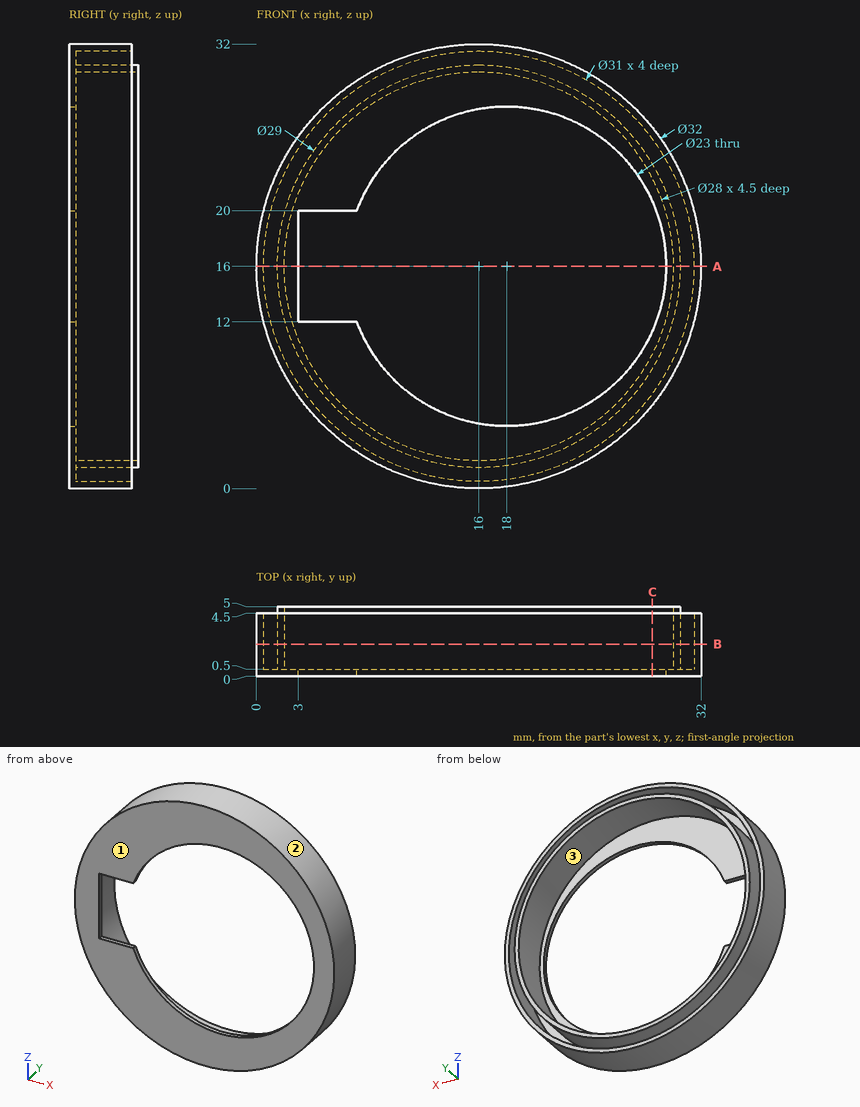
Design review of the part shown in the three views and the two pictorial views. Dimensions are in mm from the part's minimum x, y and z. Give positions to 0.01 mm unless a question says otherwise; leave off trailing zeros. Loops run counter-clockwise (first coordinate to the right, second up) from the corner with the lowest first, then second, coordinate; pieces in that order, holes last. Notation, with made-up numbers: M 12,58 L 19,58 A28 cw 19,79 Z; hole C 74,17 d5. An arc over 180 degrees is marked long. Put each result on its own line as item: value. Start each with the question number.
(1) Add section C-C, the plane x = 28.5. Write out the cut boundary in (y, z).
(2) For pin 1 (3 mm diameter, centred on x = 4, z = 19.5, fed in from -Y); pin 2 (1.5 mm diameter, centred on x = 28, y = 3.5, fed in from +Z); pin 3 (3 mm diameter, centred on y = 2.5, z = 18.5, fed in from -X), all flat-tipped, find the tip position at first contact; note any pin that passes through.
(3) Add section B-B, the plane y = 2.3. Write out the cut boundary in (x, z).
(4) The part is to be moulded in two halves that separate along Z. For the marked faces 1, 2 and 3, say which applies: +Z half, -Z half, draft (parallel to the pull), parting line (faces both ways), or undercut.
(5) Add section A-A, the plane z = 16. Write out the cut boundary in (x, y), then the cut area to 4 significant figures.
(6) Wall thickness on L1, parallel to X at y = 3.4, z = 16; L2, parallel to Z at x = 16.5, y = 0.8; L3, parallel to Z at x = 21, y = 1.55: over which ranges is each line inside the solid? List them lowest first.
Result:
1. outline: M 0,6.01 L 4.5,6.01 L 4.5,6.83 L 0.5,6.83 L 0.5,8.65 L 5,8.65 L 5,9.7 L 0.5,9.7 L 0.5,11.31 L 0,11.31 Z; M 0,20.69 L 0.5,20.69 L 0.5,22.3 L 5,22.3 L 5,23.35 L 0.5,23.35 L 0.5,25.17 L 4.5,25.17 L 4.5,25.99 L 0,25.99 Z
2. pin 1: stops at y = 0
2. pin 2: stops at z = 27.38
2. pin 3: stops at x = 0.03
3. outline: C 16,16 d32; C 16,16 d29; hole C 16,16 d31; hole C 16,16 d28
4. face 1: draft
4. face 2: parting line
4. face 3: undercut
5. outline: M 0,0 L 3,0 L 3,0.5 L 2,0.5 L 2,5 L 1.5,5 L 1.5,0.5 L 0.5,0.5 L 0.5,4.5 L 0,4.5 Z; M 29.5,0 L 32,0 L 32,4.5 L 31.5,4.5 L 31.5,0.5 L 30.5,0.5 L 30.5,5 L 30,5 L 30,0.5 L 29.5,0.5 Z
5. area: 11.25 mm^2
6. L1: x = 0 to 0.5, 1.5 to 2, 30 to 30.5, 31.5 to 32
6. L2: z = 0.01 to 0.51, 1.51 to 2.01, 29.99 to 30.49, 31.49 to 31.99
6. L3: z = 0.8 to 1.33, 2.39 to 2.92, 29.08 to 29.61, 30.67 to 31.2
